Design review of the part built by this model. Coordinates are the model's own, in mm. A direction names the side the tool comes from. Round coordinates to 2 decimals unless told otherwise and drop trailing zeros. Order: outer loops, then holes, each group sorted by start corner. A loop starts at its lowest first (then second) coordinate and runs counter-clockwise, first axis right, second up.
from build123d import *

# Parameters (mm, degrees)
PAD_DEPTH    = 26
SKETCH001_W  = 8
SKETCH001_H  = 2
POCKET_DEPTH = 2.001


with BuildPart() as part:
    # Sketch → Pad (new body)
    with BuildSketch(Plane.XZ):
        Polygon((-3.96322, 19.863666), (-3.96322, 21.863666), (-7.96322, 21.863666), (-7.96322, 9.863666), (21.2675, 9.863666), (21.2675, 21.863666), (17.2675, 21.863666), (17.2675, 19.863666), (19.2675, 19.863666), (19.2675, 17.863666), (17.2675, 17.863666), (17.2675, 11.863666), (-3.7325, 11.863666), (-3.7325, 17.863666), (-5.96322, 17.863666), (-5.96322, 19.863666), align=None)
    extrude(amount=PAD_DEPTH)

    # Sketch001 (on Face12 of Pad) → Pocket (cut, through all)
    with BuildSketch(Plane(origin=(0, 0, 11.863666), x_dir=(-1, 0, 0), z_dir=(0, 0, 1))):
        with Locations((-5.674862, 1)):
            Rectangle(SKETCH001_W, SKETCH001_H)
    extrude(amount=-POCKET_DEPTH, mode=Mode.SUBTRACT)


solid = part.part
1) For faces 1 (the face through (9.675, -1, 11)), 2 (the face through (18, -13, 19.864)), 3 (the face through (-3.963, -13, 21)), list the 3-axis set-ups (+Z, -Z, +X, -X, +Y, -Y) from which the entire face can be reached by the end or side of a thin tool; tool diameter is ignored.
Results:
face 1: +Z, -Z, +Y
face 2: +Y, -Y
face 3: +Z, +Y, -Y
2) The part is to be moulded in two halves that separate along Z. For faces 4 (the face through (7, -13, 11.864)), 5 (the face through (19.268, -13, 19)), 6 (the face through (21.268, -13, 16)), say which applies: released by +Z, released by -Z, zero draft, split by the parting line, or undercut.
Results:
face 4: released by +Z
face 5: undercut
face 6: zero draft
3) Take a section at D-D on z = 11.5. Give the boundary of the cut face in (x, y), plus the area to 3 significant figures.
Results:
outline: (-7.96, -26) - (21.27, -26) - (21.27, 0) - (9.67, 0) - (9.67, -2) - (1.67, -2) - (1.67, 0) - (-7.96, 0) - close
area: 744 mm2
4) Take a section at A-A on z = 20.75. Give the boundary of the cut face in (x, y), plus the area to 3 significant figures.
Results:
outline: (-7.96, -26) - (-3.96, -26) - (-3.96, 0) - (-7.96, 0) - close; (17.27, -26) - (21.27, -26) - (21.27, 0) - (17.27, 0) - close
area: 208 mm2
5) Take a section at C-C on y = -19.25. Give the boundary of the cut face in (x, z), plus the area to 3 significant figures.
Results:
outline: (-7.96, 9.86) - (21.27, 9.86) - (21.27, 21.86) - (17.27, 21.86) - (17.27, 19.86) - (19.27, 19.86) - (19.27, 17.86) - (17.27, 17.86) - (17.27, 11.86) - (-3.73, 11.86) - (-3.73, 17.86) - (-5.96, 17.86) - (-5.96, 19.86) - (-3.96, 19.86) - (-3.96, 21.86) - (-7.96, 21.86) - close
area: 132 mm2
6) To check wall thickness, follow line 1 along X through (y, z) = (-18.5, 18); line 2 along X through (y, z) = (-8.75, 17.25); line 3 along Z through (x, y) = (17.5, -21.75). State the ranges of each line that lie inside material, in increasing order.
Results:
line 1: x = -7.96 to -5.96, 19.27 to 21.27
line 2: x = -7.96 to -3.73, 17.27 to 21.27
line 3: z = 9.86 to 17.86, 19.86 to 21.86
7) Clearance check with flat-ended pins moving along their axes: P1, Ø2, axis at x = 3, y = -21.5, coming from the +Z side; P2, Ø1, axis at x = 4, z = 10.5, coming from the +Y side; P3, Ø8, axis at x = 15.5, y = -14, coming from the +Z side. State where each tip first meets the part, or that it passes through.
Results:
P1: stops at z = 11.86
P2: stops at y = -2
P3: stops at z = 21.86
8) Take a section at B-B on x = -4.5. Give the boundary of the cut face in (y, z).
Results:
outline: (-26, 9.86) - (0, 9.86) - (0, 17.86) - (-26, 17.86) - close; (-26, 19.86) - (0, 19.86) - (0, 21.86) - (-26, 21.86) - close
